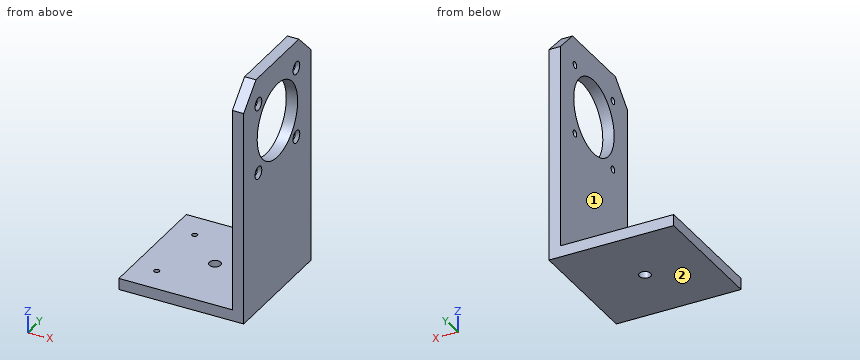
```python
from build123d import *

# Parameters (mm, degrees)
SKETCH1_W                                         = 55
SKETCH1_H                                         = 55
BOSS_EXTRUDE1_DEPTH                               = 5
SKETCH2_W                                         = 5
SKETCH2_H                                         = 55
BOSS_EXTRUDE2_DEPTH                               = 100
CUT_EXTRUDE1_REACH                                = 57
SKETCH3_R                                         = 16.5
CUT_EXTRUDE2_REACH                                = 7
SKETCH4_R                                         = 2.5
CUT_EXTRUDE3_REACH                                = 57
F_4_48_TAPPED_HOLE1_D                             = 2.3749
F_4_48_TAPPED_HOLE1_DEPTH                         = 3.5
F_4_48_TAPPED_HOLE1_TIP                           = 0.713491942
CSK_FOR_M2_5_FLAT_HEAD_MACHINE_SCREW1_D           = 2.9
CSK_FOR_M2_5_FLAT_HEAD_MACHINE_SCREW1_DEPTH       = 5
CSK_FOR_M2_5_FLAT_HEAD_MACHINE_SCREW1_CSINK_D     = 5.5
CSK_FOR_M2_5_FLAT_HEAD_MACHINE_SCREW1_CSINK_ANGLE = 90


with BuildPart() as part:
    # Sketch1 → Boss-Extrude1 (new body)
    with BuildSketch(Plane.XY):
        Rectangle(SKETCH1_W, SKETCH1_H)
    extrude(amount=BOSS_EXTRUDE1_DEPTH)

    # Sketch2 → Boss-Extrude2 (add)
    with BuildSketch(Plane.XY.offset(5)):
        with Locations((25, 0)):
            Rectangle(SKETCH2_W, SKETCH2_H)
    extrude(amount=BOSS_EXTRUDE2_DEPTH)

    # Sketch3 → Cut-Extrude1 (cut, up to next)
    with BuildSketch(Plane(origin=(27.5, 0, 0), x_dir=(0, 0, -1), z_dir=(1, 0, 0)), mode=Mode.PRIVATE) as cut_extrude1_sk1:
        with Locations((-77.5, 0)):
            Circle(SKETCH3_R)
    cut_extrude1_tool1 = extrude(cut_extrude1_sk1.sketch, amount=-CUT_EXTRUDE1_REACH, mode=Mode.PRIVATE) & part.part
    add(cut_extrude1_tool1.solids().sort_by_distance((27.5, 0, 77.5))[0], mode=Mode.SUBTRACT)

    # Sketch4 → Cut-Extrude2 (cut, up to next)
    with BuildSketch(Plane.XY.offset(5), mode=Mode.PRIVATE) as cut_extrude2_sk1:
        Circle(SKETCH4_R)
    cut_extrude2_tool1 = extrude(cut_extrude2_sk1.sketch, amount=-CUT_EXTRUDE2_REACH, mode=Mode.PRIVATE) & part.part
    add(cut_extrude2_tool1.solids().sort_by_distance((0, 0, 5))[0], mode=Mode.SUBTRACT)

    # Sketch5 → Cut-Extrude3 (cut, up to next)
    with BuildSketch(Plane(origin=(27.5, 0, 0), x_dir=(0, 0, -1), z_dir=(1, 0, 0)), mode=Mode.PRIVATE) as cut_extrude3_sk1:
        Polygon((-105, 27.5), (-95, 27.5), (-105, 17.5), align=None)
    cut_extrude3_tool1 = extrude(cut_extrude3_sk1.sketch, amount=-CUT_EXTRUDE3_REACH, mode=Mode.PRIVATE) & part.part
    add(cut_extrude3_tool1.solids().sort_by_distance((27.5, 24.166667, 101.666667))[0], mode=Mode.SUBTRACT)
    # Sketch5 → Cut-Extrude3 (cut, up to next)
    with BuildSketch(Plane(origin=(27.5, 0, 0), x_dir=(0, 0, -1), z_dir=(1, 0, 0)), mode=Mode.PRIVATE) as cut_extrude3_sk2:
        Polygon((-105, -27.5), (-95, -27.5), (-105, -17.5), align=None)
    cut_extrude3_tool2 = extrude(cut_extrude3_sk2.sketch, amount=-CUT_EXTRUDE3_REACH, mode=Mode.PRIVATE) & part.part
    add(cut_extrude3_tool2.solids().sort_by_distance((27.5, -24.166667, 101.666667))[0], mode=Mode.SUBTRACT)

    # #4-48 Tapped Hole1
    with Locations(Plane.XY.offset(5)):
        with Locations((-17.3, 15.5), (-17.3, -15.5)):
            Hole(F_4_48_TAPPED_HOLE1_D / 2, depth=F_4_48_TAPPED_HOLE1_DEPTH)
            with Locations((0, 0, -(F_4_48_TAPPED_HOLE1_DEPTH + F_4_48_TAPPED_HOLE1_TIP / 2))):  # 118° drill point
                Cone(0, F_4_48_TAPPED_HOLE1_D / 2, F_4_48_TAPPED_HOLE1_TIP, mode=Mode.SUBTRACT)

    # CSK for M2.5 Flat Head Machine Screw1
    with Locations(Plane(origin=(27.5, 0, 0), x_dir=(0, 0, -1), z_dir=(1, 0, 0))):
        with Locations((-93, 15.5), (-62, 15.5), (-62, -15.5), (-93, -15.5)):
            CounterSinkHole(CSK_FOR_M2_5_FLAT_HEAD_MACHINE_SCREW1_D / 2, CSK_FOR_M2_5_FLAT_HEAD_MACHINE_SCREW1_CSINK_D / 2, depth=CSK_FOR_M2_5_FLAT_HEAD_MACHINE_SCREW1_DEPTH, counter_sink_angle=CSK_FOR_M2_5_FLAT_HEAD_MACHINE_SCREW1_CSINK_ANGLE)


solid = part.part
```
Model file for the job. Use its own axes, mm. Face numbers are marked on the shaded views. A direction names the side the tool comes from. Coordinates: 2 decimals unless noted, no trailing zeros. Order: outer loops, then holes, each group sorted by start corner. A loop starts at its lowest first (then second) coordinate and runs counter-clockwise, first axis right, second up. Notation, with made-up numbers: (30.5, 16) -> (58.5, 16) arc R16 ccw to (58.5, 25) -> close; hole circle Ø11 at (47, 2). An arc over 180 degrees is marked (long way). Answer as a JSON object with one key per item and string values. Group by question number.
1) Cut at C-C, the plane y = 6.5. Write the cut outline in (x, z), then the cut area to 3 significant figures.
2) Flat gauge pins, fed straight in: pin 1 (3.5 mm diameter, centred on y = 15.5, z = 62, fed in from -X); pin 2 (1.7 mm diameter, centred on y = -15.5, z = 93, fed in from -X); pin 3 (4 mm diameter, centred on x = -11.5, y = -8, fed in from +Z); pin 4 (4.5 mm diameter, centred on y = 15.5, z = 93, fed in from +X). Where does each tip first touch, or does it go through?
3) Cut at B-B, the plane z = 70.5. Write the cut outline in (x, y).
4) Cut at A-A, the plane x = 0. Write the cut outline in (y, z), then the cut area to 3 significant figures.
5) Drill centre lines: L1, parallel to Y at x = -17.3, z = 2.75; L2, parallel to Z at x = 25, y = -15; L3, parallel to Y at x = -17, z = 4. Where is each one in solid material? Low to high.
6) Cut at D-D, the plane x = 8.5. Write the cut outline in (y, z).
7) Which spindle directions (+Z, -Z, +X, -X, +Y, -Y) get a long thin tool onto all of the face, cutting with end or side? Do the marked faces 1 and 2. Say none if no direction does.
Check values:
{
 "1": {"outline": "(-27.5, 0) -> (27.5, 0) -> (27.5, 62.33) -> (22.5, 62.33) -> (22.5, 5) -> (-27.5, 5) -> close; (22.5, 92.67) -> (27.5, 92.67) -> (27.5, 105) -> (22.5, 105) -> close", "area": "623 mm²"},
 "2": {"pin 1": "stops at x = 22.5", "pin 2": "passes through", "pin 3": "stops at z = 5", "pin 4": "stops at x = 27"},
 "3": {"outline": "(22.5, -27.5) -> (27.5, -27.5) -> (27.5, -14.94) -> (22.5, -14.94) -> close; (22.5, 14.94) -> (27.5, 14.94) -> (27.5, 27.5) -> (22.5, 27.5) -> close"},
 "4": {"outline": "(-27.5, 0) -> (-2.5, 0) -> (-2.5, 5) -> (-27.5, 5) -> close; (2.5, 0) -> (27.5, 0) -> (27.5, 5) -> (2.5, 5) -> close", "area": "250 mm²"},
 "5": {"L1": "y = -27.5 to -16.69, -14.31 to 14.31, 16.69 to 27.5", "L2": "z = 0 to 60.64, 63.36 to 70.63, 84.37 to 91.64, 94.36 to 105", "L3": "y = -27.5 to -16.65, -14.35 to 14.35, 16.65 to 27.5"},
 "6": {"outline": "(-27.5, 0) -> (27.5, 0) -> (27.5, 5) -> (-27.5, 5) -> close"},
 "7": {"face 1": "+Z, -X, +Y, -Y", "face 2": "-Z, +X, -X, +Y, -Y"}
}
